Geometry: final body of the model. Coordinates: model frame, mm. Face numbers are marked on the shaded views. Coordinates: 2 decimals unless noted, no trailing zeros. Return JSON: item names as keys, results as strings.
from build123d import *

# Parameters (mm, degrees)
SKETCH1_R           = 55
BOSS_EXTRUDE1_DEPTH = 50
SKETCH2_R           = 50
CUT_EXTRUDE1_DEPTH  = 48
CUT_EXTRUDE2_DEPTH  = 64
SKETCH4_R           = 45
BOSS_EXTRUDE2_DEPTH = 2
FILLET1_R           = 8


with BuildPart() as part:
    # Sketch1 → Boss-Extrude1 (new body)
    with BuildSketch(Plane(origin=(0, 0, 0), x_dir=(1, 0, 0), z_dir=(0, 1, 0))):
        Circle(SKETCH1_R)
    extrude(amount=BOSS_EXTRUDE1_DEPTH)

    # Sketch2 → Cut-Extrude1 (cut)
    with BuildSketch(Plane(origin=(0, 50, 0), x_dir=(1, 0, 0), z_dir=(0, 1, 0))):
        Circle(SKETCH2_R)
    extrude(amount=-CUT_EXTRUDE1_DEPTH, mode=Mode.SUBTRACT)

    # Sketch3 → Cut-Extrude2 (cut, symmetric)
    with BuildSketch(Plane(origin=(0, 0, 0), x_dir=(0, 0, -1), z_dir=(1, 0, 0))):
        with BuildLine():
            Line((-55, 10), (-55, 50))
            Line((-55, 50), (55, 50))
            add(Edge.make_bspline(
                [(-55, 10), (-32.185575053, 27.405291441), (13.190680472, 18.202995652), (46.289902957, 40.289555955), (55, 50)],
                knots=[0, 0, 0, 0, 0.690633178, 1, 1, 1, 1], degree=3))
        make_face()
    extrude(amount=CUT_EXTRUDE2_DEPTH, both=True, mode=Mode.SUBTRACT)

    # Sketch4 → Boss-Extrude2 (add)
    with BuildSketch(Plane.XZ):
        Circle(SKETCH4_R)
    extrude(amount=BOSS_EXTRUDE2_DEPTH)

    # Fillet1
    fillet1_edges = [part.edges().sort_by_distance(p)[0] for p in [
        (-55, 0, 0),
    ]]
    fillet(fillet1_edges, radius=FILLET1_R)


solid = part.part
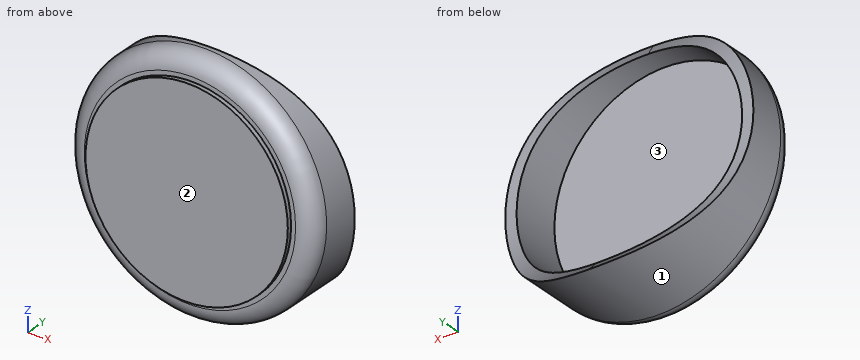
Item 1: First-contact query: pin 1 Ø3 at (x, y) = (31.5, 36) entering from +Z; pin 2 Ø5 at (x, z) = (35.5, -36.5) entering from -Y; pin 3 Ø12 at (x, y) = (-32.5, 11.5) entering from +Z. Flat tips, straight axial feed; report the tip coordinate or a pass-through.
Worked out:
{"pin 1": "z = -37.62", "pin 2": "y = 0.13", "pin 3": "z = 48.19"}
Item 2: Mould query, pull axis X, two halves, no side actions, for the marked faces 1, 2 and 3. Classes: +X half, -X half, draft (parallel to the pull), parting line (faces both ways), or undercut.
Worked out:
{"face 1": "parting line", "face 2": "draft", "face 3": "undercut"}
Item 3: Ray query, probe 1 along X at (y, z) = (12, 0); probe 2 along Y at (x, z) = (-10, -0.5); probe 3 along Z at (x, y) = (0, 36). Return the intervals inside material, ascending. Write a range as from..to.
Worked out:
{"probe 1": "-55..-50, 50..55", "probe 2": "-2..2", "probe 3": "-55..-50"}
